Autodesk Inventor part; units mm, degrees
ref_plane "工作平面1" through (0, 0, 50) normal (0, 0, -1) x (-1, 0, 0)
ref_plane "YZ Plane" through (0, 0, 0) normal (1, 0, 0) x (0, 1, 0)
ref_plane "XZ Plane" through (0, 0, 0) normal (0, 1, 0) x (-1, 0, 0)
sketch "草图1" plane through (0, 0, 0) normal (0, 0, 1) x (1, 0, 0)
  line L0 (27.5, -10) -> (-27.5, -10)
  line L1 (-27.5, -10) -> (-27.5, 10)
  line L2 (-27.5, 10) -> (27.5, 10)
  line L3 (27.5, 10) -> (27.5, -10)
  line L4 (27.5, -10) -> (-27.5, 10) construction
  line L5 (-27.5, -10) -> (27.5, 10) construction
  point P0 (0, 0)
  dimension "d0" = 55
  dimension "d1" = 20
extrude "拉伸1" add sketch "草图1" along normal blind 100
sketch "草图2" plane through (0, 0, 0) normal (0, 0, -1) x (-1, 0, 0)
  line L0 (-27.5, 10) -> (27.5, 10)
  line L1 (-27.5, -10) -> (-27.5, 10)
  line L2 (27.5, -10) -> (-27.5, -10)
  line L3 (27.5, 10) -> (27.5, -10)
  line L4 (26.5, -9) -> (-26.5, -9)
  line L5 (-26.5, -9) -> (-26.5, 9)
  line L6 (-26.5, 9) -> (26.5, 9)
  line L7 (26.5, 9) -> (26.5, -9)
  point P0 (0, 0)
  dimension "d4" = 1
extrude "拉伸2" cut sketch "草图2" against normal blind 109.25 contours L4 L5 L6 L7
sketch "草图3" plane through (-27.5, -10, 0) normal (-1, 0, 0) x (0, 0, 1)
  line L0 (100, 19) -> (100, 1)
  line L1 (100, 10) -> (53.3489, 10)
  circle A0 centre (93.6894, 10) radius 3
  point P0 (0, 10)
  dimension "d7" = 6
extrude "拉伸3" cut sketch "草图3" against normal blind 109.25
ref_plane "工作平面1" through (0, 0, 50) normal (0, 0, -1) x (-1, 0, 0)
mirror "镜像1" about plane through (0, 0, 50) normal (0, 0, -1) of "拉伸3"
sketch "草图4" plane through (-27.5, 10, 0) normal (0, 1, 0) x (1, 0, 0)
  line L0 (54, 0) -> (54, -100)
  line L1 (55, 0) -> (55, -100)
  circle A0 centre (232, -40) radius 2.5
  circle A1 centre (40, -60) radius 2.5
  circle A2 centre (212, -40) radius 2.5
  circle A3 centre (212, -60) radius 2.5
  circle A4 centre (20, -40) radius 2.5
  circle A5 centre (20, -60) radius 2.5
  circle A6 centre (232, -60) radius 2.5
  circle A7 centre (40, -40) radius 2.5
  line L2 (61, -70) -> (61, -150)
  line L3 (61, -150) -> (191, -150)
  line L4 (191, -150) -> (191, -70)
  line L5 (191, -70) -> (246, -70)
  line L6 (246, -70) -> (246, -30)
  line L7 (246, -30) -> (191, -30)
  line L8 (191, -30) -> (191, 50)
  line L9 (191, 50) -> (61, 50)
  line L10 (61, 50) -> (61, -30)
  line L11 (61, -30) -> (6, -30)
  line L12 (6, -30) -> (6, -70)
  line L13 (6, -70) -> (61, -70)
  point P0 (27.5, 0)
extrude "拉伸4" cut sketch "草图4" against normal blind 42.75 contours A1 | A4 | A5 | A7
properties part number "铝方管"
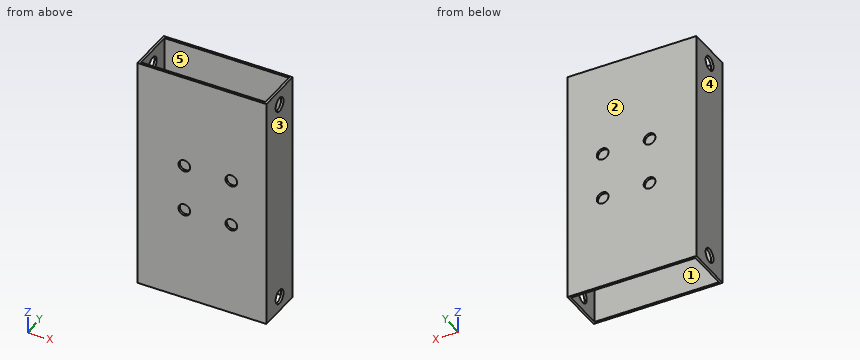
Work out the finished part from the listing and answer in its coordinate system (mm). Face numbers are marked on the shaded views. A direction names the side the tool comes from. Give positions to 0.01 mm unless a question says otherwise; leave off trailing zeros. Write each loop counter-clockwise with the first axis right and the second up, starting at its lowest first coordinate (ties: lowest second). Pieces come first, ordered by that corner, then holes.
(1) The part is cut by section A-A on x = 12.5. Write down the section's boundary in (y, z), plus the area to 3 significant figures.
Final values:
outline: (-10, 0) - (-9, 0) - (-9, 37.5) - (-10, 37.5) - close; (-10, 42.5) - (-9, 42.5) - (-9, 57.5) - (-10, 57.5) - close; (-10, 62.5) - (-9, 62.5) - (-9, 100) - (-10, 100) - close; (9, 0) - (10, 0) - (10, 37.5) - (9, 37.5) - close; (9, 42.5) - (10, 42.5) - (10, 57.5) - (9, 57.5) - close; (9, 62.5) - (10, 62.5) - (10, 100) - (9, 100) - close
area: 180 mm2
(2) The part is cut by section C-C on y = 8. Write down the section's boundary in (x, z), plus the area to 3 significant figures.
Final values:
outline: (-27.5, 0) - (-26.5, 0) - (-26.5, 100) - (-27.5, 100) - close; (26.5, 0) - (27.5, 0) - (27.5, 100) - (26.5, 100) - close
area: 200 mm2
(3) The mould has two halves that part along X. Classify the marked faces 1, 2 and 3: pulls with the +X half, pulls with the -X half, needs draft (parallel to the pull), parting line crosses it, or undercut.
Final values:
face 1: undercut
face 2: needs draft
face 3: pulls with the +X half
(4) Which of the six approach directions +Z, -Z, +X, -X, +Y, -Y give full straight-line access (tool end or side, diameter ignored) to the marked faces 4 and 5?
Final values:
face 4: +Z, -Z, -X, +Y, -Y
face 5: +Z, -Z
(5) The part is cut by section D-D on z = 60. Write down the section's boundary in (x, y).
Final values:
outline: (-27.5, -10) - (-10, -10) - (-10, -9) - (-26.5, -9) - (-26.5, 9) - (-10, 9) - (-10, 10) - (-27.5, 10) - close; (-5, -10) - (10, -10) - (10, -9) - (-5, -9) - close; (-5, 9) - (10, 9) - (10, 10) - (-5, 10) - close; (15, -10) - (27.5, -10) - (27.5, 10) - (15, 10) - (15, 9) - (26.5, 9) - (26.5, -9) - (15, -9) - close
(6) The part is cut by section B-B on z = 88.5. Write down the section's boundary in (x, y).
Final values:
outline: (-27.5, -10) - (27.5, -10) - (27.5, 10) - (-27.5, 10) - close; hole (-26.5, -9) - (26.5, -9) - (26.5, 9) - (-26.5, 9) - close
(7) Straight lines are drawn through the part: line 1 (X direction, y = 9.4, z = 60); line 2 (Z direction, x = 12.5, y = -9.65); line 3 (X direction, y = 3.75, z = 38). For each, find the intervals that lie inside material, in ascending order.
Final values:
line 1: x = -27.5 to -10, -5 to 10, 15 to 27.5
line 2: z = 0 to 37.5, 42.5 to 57.5, 62.5 to 100
line 3: x = -27.5 to -26.5, 26.5 to 27.5
